Source: CAD feature listing. Evaluate the final solid. Frame: model axes, mm. Round coordinates to 2 decimals unless told otherwise and drop trailing zeros. Loops run counter-clockwise (first coordinate to the right, second up) from the corner with the lowest first, then second, coordinate; pieces in that order, holes last.
(1) First-contact query: pin 1 Ø0.9 at (x, z) = (15, 2) entering from +Y; pin 2 Ø3.5 at (x, y) = (15.25, 13) entering from +Z; pin 3 Ø0.9 at (y, z) = (35, 1.5) entering from -X. Flat tips, straight axial feed; report the tip coordinate or a pass-through.
(2) Section C-C, the plane y = -1. Return the cut outline in (x, z).
(3) Section B-B, the plane z = 2. Count the separate pieces of the cut face and the enclosed holes in it, plus the area to 3 significant figures.
(4) Material intervals for probe 1 along Y at (x, z) = (15.25, 1.8); probe 2 along X at (y, z) = (22, 0.7); probe 3 along X at (y, z) = (9, 1.8), sorted ascending.
(5) Section A-A, the plane x = 15.25. Return the cut outline in (y, z), plus the area to 3 significant figures.
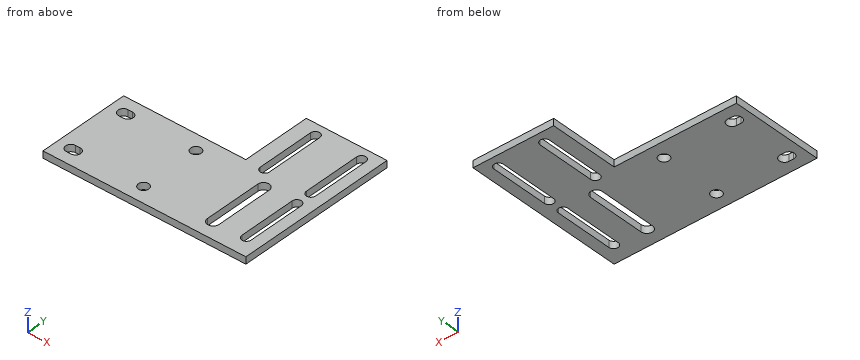
```python
from build123d import *

# Parameters (mm, degrees)
SKETCH_1_R      = 2.25
EXTRUDE_1_DEPTH = 3


with BuildPart() as part:
    # 草图1 → 凸台-拉伸1 (new body)
    with BuildSketch(Plane.XY):
        Polygon((65.75, -20), (-22.25, -20), (-22.25, 20), (30.75, 20), (30.75, 50), (65.75, 50), (65.75, 20), align=None)
        with Locations((15.25, 13)):
            Circle(SKETCH_1_R, mode=Mode.SUBTRACT)
        with Locations((15.25, -13)):
            Circle(SKETCH_1_R, mode=Mode.SUBTRACT)
        with BuildLine():
            Line((-14.25, 10.75), (-16.25, 10.75))
            ThreePointArc((-16.25, 10.75), (-18.5, 13), (-16.25, 15.25))
            Line((-16.25, 15.25), (-14.25, 15.25))
            ThreePointArc((-14.25, 15.25), (-12, 13), (-14.25, 10.75))
        make_face(mode=Mode.SUBTRACT)
        with BuildLine():
            Line((-14.25, -15.25), (-16.25, -15.25))
            ThreePointArc((-16.25, -15.25), (-18.5, -13), (-16.25, -10.75))
            Line((-16.25, -10.75), (-14.25, -10.75))
            ThreePointArc((-14.25, -10.75), (-12, -13), (-14.25, -15.25))
        make_face(mode=Mode.SUBTRACT)
        with BuildLine():
            Line((42.5, -12.5), (42.5, 12.5))
            ThreePointArc((42.5, 12.5), (45, 15), (47.5, 12.5))
            Line((47.5, 12.5), (47.5, -12.5))
            ThreePointArc((47.5, -12.5), (45, -15), (42.5, -12.5))
        make_face(mode=Mode.SUBTRACT)
        with BuildLine():
            Line((57, 20), (57, 45))
            ThreePointArc((57, 45), (59, 47), (61, 45))
            Line((61, 45), (61, 20))
            ThreePointArc((61, 20), (59, 18), (57, 20))
        make_face(mode=Mode.SUBTRACT)
        with BuildLine():
            Line((61, -12), (61, 13))
            ThreePointArc((61, 13), (59, 15), (57, 13))
            Line((57, 13), (57, -12))
            ThreePointArc((57, -12), (59, -14), (61, -12))
        make_face(mode=Mode.SUBTRACT)
        with BuildLine():
            Line((41, 20), (41, 45))
            ThreePointArc((41, 45), (39, 47), (37, 45))
            Line((37, 45), (37, 20))
            ThreePointArc((37, 20), (39, 18), (41, 20))
        make_face(mode=Mode.SUBTRACT)
    extrude(amount=EXTRUDE_1_DEPTH)


solid = part.part
```
Output values:
1. pin 1: stops at y = 20
1. pin 2: passes through
1. pin 3: stops at x = 30.75
2. outline: (-22.25, 0) - (42.5, 0) - (42.5, 3) - (-22.25, 3) - close; (47.5, 0) - (57, 0) - (57, 3) - (47.5, 3) - close; (61, 0) - (65.75, 0) - (65.75, 3) - (61, 3) - close
3. separate pieces: 1
3. enclosed holes: 8
3. area: 4,010 mm2
4. probe 1: y = -20 to -15.25, -10.75 to 10.75, 15.25 to 20
4. probe 2: x = 30.75 to 37, 41 to 57, 61 to 65.75
4. probe 3: x = -22.25 to 42.5, 47.5 to 57, 61 to 65.75
5. outline: (-20, 0) - (-15.25, 0) - (-15.25, 3) - (-20, 3) - close; (-10.75, 0) - (10.75, 0) - (10.75, 3) - (-10.75, 3) - close; (15.25, 0) - (20, 0) - (20, 3) - (15.25, 3) - close
5. area: 93.0 mm2
